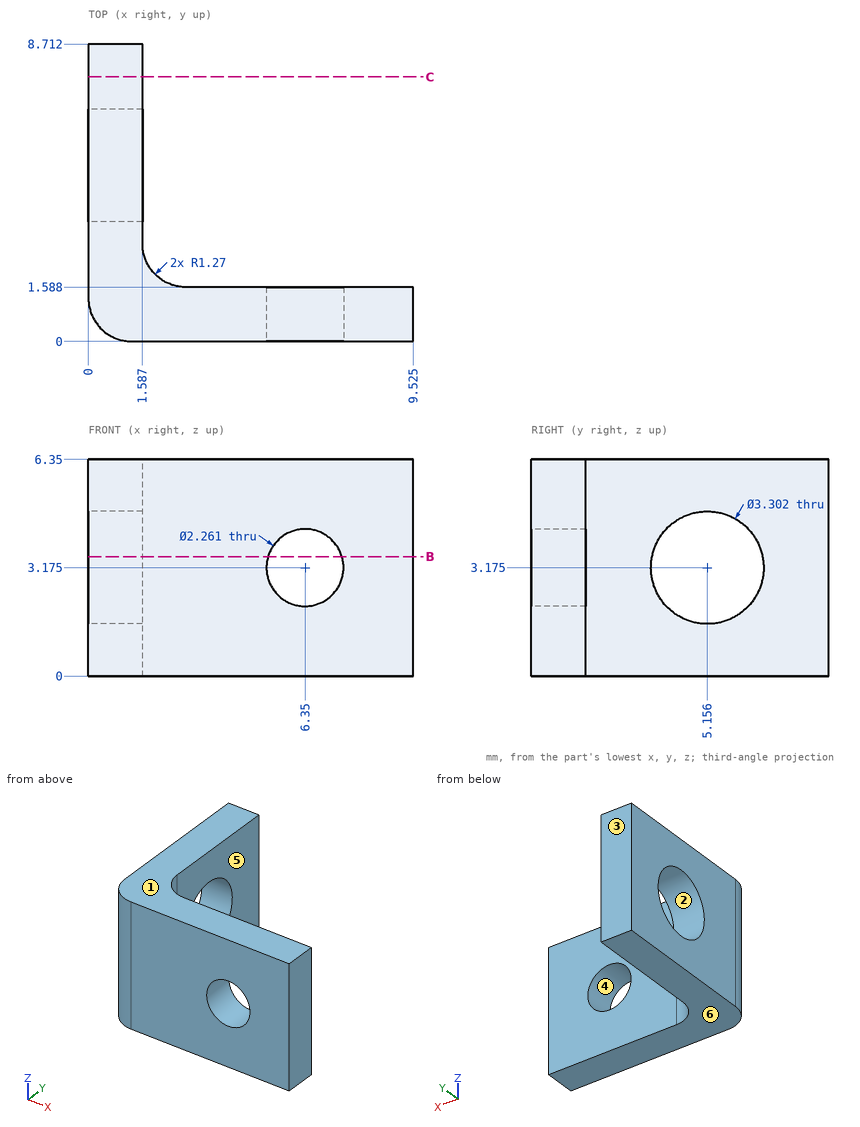
Source: three-view drawing plus pictorial views. Frame: mm from the lowest corner of the part. A direction names the side the tool comes from. Round coordinates to 2 decimals unless told otherwise and drop trailing zeros. Order: outer loops, then holes, each group sorted by start corner. A loop starts at its lowest first (then second) coordinate and runs counter-clockwise, first axis right, second up. Notation, with made-up numbers: (22, -25.5) - (48, -25.5) arc R35 cw to (48, 11.5) - close; hole circle Ø5 at (73, 79). An arc over 180 degrees is marked (long way). Answer in a Markdown table with one row per item.
Item 1: Pin query (flat end, axial travel): pin 1 (3 mm diameter, centred on x = 8, z = 3, fed in from +Y). Return the tip coordinate at first contact, or that it passes through.
Model answer:
| item | result |
|---|---|
| pin 1 | stops at y = 1.59 |
Item 2: Section query C-C (y = 7.75). Return the cut outline in (x, z), then the cut area to 3 significant figures.
Model answer:
| item | result |
|---|---|
| outline | (0, 0) - (1.59, 0) - (1.59, 6.35) - (0, 6.35) - close |
| area | 10.1 mm² |
Item 3: Line query: line 1 (Y direction, x = 5, z = 0.5); line 2 (X direction, y = 0.5, z = 2.25) (1 decimal). Output: solid intervals per line, ascending.
Model answer:
| item | result |
|---|---|
| line 1 | y = 0 to 1.59 |
| line 2 | x = 0.3 to 5.7, 7 to 9.5 |
Item 4: Mould query, pull axis Z, two halves, no side actions, for the marked faces 1, 2, 3 and 4. Classes: released by +Z, released by -Z, zero draft, split by the parting line, or undercut.
Model answer:
| item | result |
|---|---|
| face 1 | released by +Z |
| face 2 | undercut |
| face 3 | zero draft |
| face 4 | undercut |
Item 5: Reachability of the marked faces 5 and 6 from +Z, -Z, +X, -X, +Y, -Y: full face, straight path, thin tool, end or side. Return the list, or none.
Model answer:
| item | result |
|---|---|
| face 5 | +Z, -Z, +X, +Y |
| face 6 | -Z, +X, -X, +Y, -Y |
Item 6: Section query B-B (z = 3.5). Return the cut outline in (x, y) (1 decimal).
Model answer:
| item | result |
|---|---|
| outline | (0, 1.3) arc R1.3 ccw to (1.3, 0) - (5.3, 0) - (5.3, 1.6) - (2.9, 1.6) arc R1.3 cw to (1.6, 2.9) - (1.6, 3.5) - (0, 3.5) - close; (0, 6.8) - (1.6, 6.8) - (1.6, 8.7) - (0, 8.7) - close; (7.4, 0) - (9.5, 0) - (9.5, 1.6) - (7.4, 1.6) - close |
